The listing builds one solid part. Answer for the finished solid, in the listing's coordinates (mm). A direction names the side the tool comes from. Give positions to 0.01 mm unless a question says otherwise; leave off trailing zeros. Order: outer loops, then holes, each group sorted by start corner. A loop starts at its lowest first (then second) coordinate and runs counter-clockwise, first axis right, second up. Notation, with made-up numbers: (43, 85) - (90, 85) arc R15 cw to (90, 96) - close; hole circle Ø10 at (-14.75, 7.5). An arc over 180 degrees is marked (long way). Answer in a Markdown table with one row per item.
from build123d import *

# Parameters (mm, degrees)
SKETCH073_W             = 75.5
SKETCH073_H             = 44
PAD038_DEPTH            = 1
SKETCH074_W             = 15
SKETCH074_H             = 44
PAD039_DEPTH            = 9
SKETCH075_W             = 18
SKETCH075_H             = 44
PAD040_DEPTH            = 1
SKETCH076_W             = 10.5
SKETCH076_H             = 39.5
PAD041_DEPTH            = 30.5
SKETCH077_W             = 7
SKETCH077_H             = 30
POCKET027_DEPTH         = 39
SKETCH078_W             = 15
SKETCH078_H             = 6
POCKET028_DEPTH         = 15
SKETCH079_W             = 1.5
SKETCH079_H             = 44
PAD042_DEPTH            = 2
CHAMFER044_SIZE         = 1.2
FILLET011_R             = 7.5
CHAMFER045_SIZE         = 0.5
CHAMFER050_SIZE         = 0.3
BODY014_PLACEMENT_ANGLE = 180


with BuildPart() as part:
    # Sketch073 → Pad038 (new body)
    with BuildSketch(Plane.XY):
        with Locations((-30.25, 0)):
            Rectangle(SKETCH073_W, SKETCH073_H)
    extrude(amount=-PAD038_DEPTH)

    # Sketch074 (on Face5 of Pad038) → Pad039 (join)
    with BuildSketch(Plane.XY):
        Rectangle(SKETCH074_W, SKETCH074_H)
    extrude(amount=PAD039_DEPTH)

    # Sketch075 (on Face5 of Pad039) → Pad040 (join)
    with BuildSketch(Plane.XY.offset(9)):
        with Locations((-1.5, 0)):
            Rectangle(SKETCH075_W, SKETCH075_H)
    extrude(amount=PAD040_DEPTH)

    # Sketch076 (on Face7 of Pad040) → Pad041 (join)
    with BuildSketch(Plane.XY.offset(10)):
        Rectangle(SKETCH076_W, SKETCH076_H)
    extrude(amount=PAD041_DEPTH)

    # Sketch077 (on Face15 of Pad041) → Pocket027 (cut)
    with BuildSketch(Plane.XY.offset(40.5)):
        Rectangle(SKETCH077_W, SKETCH077_H)
    extrude(amount=-POCKET027_DEPTH, mode=Mode.SUBTRACT)

    # Sketch078 (on Face6 of Pocket027) → Pocket028 (cut)
    with BuildSketch(Plane.YZ.offset(7.5)):
        with Locations((0, 4.5)):
            Rectangle(SKETCH078_W, SKETCH078_H)
    extrude(amount=-POCKET028_DEPTH, mode=Mode.SUBTRACT)

    # Sketch079 (on Face4 of Pocket028) → Pad042 (join)
    with BuildSketch(Plane.XY):
        with Locations((-61.25, 0)):
            Rectangle(SKETCH079_W, SKETCH079_H)
    extrude(amount=PAD042_DEPTH)

    # Chamfer044
    chamfer044_edges = [part.edges().sort_by_distance(p)[0] for p in [
        (-62, 0, 2),
    ]]
    chamfer(chamfer044_edges, length=CHAMFER044_SIZE)

    # Fillet011
    fillet011_edges = [part.edges().sort_by_distance(p)[0] for p in [
        (0, 15, 1.5),
        (0, -15, 1.5),
    ]]
    fillet(fillet011_edges, radius=FILLET011_R)

    # Chamfer045
    chamfer045_edges = [part.edges().sort_by_distance(p)[0] for p in [
        (-7.5, 7.5, 4.5),
        (-7.5, 0, 7.5),
        (-7.5, -7.5, 4.5),
        (-7.5, 0, 1.5),
        (7.5, 7.5, 4.5),
        (7.5, 0, 1.5),
        (7.5, -7.5, 4.5),
        (7.5, 0, 7.5),
        (7.5, -22, 4.5),
        (7.5, 22, 4.5),
        (7.5, 0, -1),
        (-7.5, -22, 4.5),
        (-30.25, -22, -1),
        (-68, 0, -1),
        (-30.25, 22, -1),
        (-7.5, 22, 4.5),
        (-10.5, -22, 9.5),
        (-10.5, 22, 9.5),
    ]]
    chamfer(chamfer045_edges, length=CHAMFER045_SIZE)

    # Chamfer050
    chamfer050_edges = [part.edges().sort_by_distance(p)[0] for p in [
        (5.25, 19.75, 25.25),
        (-5.25, 19.75, 25.25),
        (-5.25, -19.75, 25.25),
        (5.25, -19.75, 25.25),
        (0, 19.75, 40.5),
        (-5.25, 0, 40.5),
        (5.25, 0, 40.5),
        (0, -19.75, 40.5),
        (-3.5, 0, 40.5),
        (0, -15, 40.5),
        (3.5, 0, 40.5),
        (0, 15, 40.5),
    ]]
    chamfer(chamfer050_edges, length=CHAMFER050_SIZE)


with BuildPart() as part_1:
    # Body014 placement: moved
    add(part.part.moved(Location((-106.5, -22, -136))).rotate(Axis((-106.5, -22, -136), (0, 0, 1)), BODY014_PLACEMENT_ANGLE))


solid = part_1.part
Item 1: Determine the mould class of faces 1 (the face through (-101.25, -22, -111)), 2 (the face through (-101, 0, -132)), 3 (the face through (-46, -22, -135)) for opening direction X: pulls with the +X half, pulls with the -X half, needs draft (parallel to the pull), parting line crosses it, or undercut.
Answer block:
| item | result |
|---|---|
| face 1 | pulls with the +X half |
| face 2 | needs draft |
| face 3 | undercut |
Item 2: Find section A-A on z = -99. Write down the section's boundary in (x, y), then the cut area to 3 significant figures.
Answer block:
| item | result |
|---|---|
| outline | (-111.75, -41.45) - (-111.45, -41.75) - (-101.55, -41.75) - (-101.25, -41.45) - (-101.25, -2.55) - (-101.55, -2.25) - (-111.45, -2.25) - (-111.75, -2.55) - close; hole (-110, -37) - (-103, -37) - (-103, -7) - (-110, -7) - close |
| area | 205 mm² |
Item 3: Consider line 1 (Y direction, x = -106.5, z = -117); line 2 (X direction, y = -25.5, z = -125); line 3 (Z direction, x = -54.5, y = -8). Determine where each line is inside the solid, lowest interval first.
Answer block:
| item | result |
|---|---|
| line 1 | -41.75 to -37, -7 to -2.25 |
| line 2 | -111.75 to -110, -103 to -101.25 |
| line 3 | -137 to -136 |
Item 4: Find section D-D on y = -40. Write down the section's boundary in (x, z), then the cut area to 3 significant figures.
Answer block:
| item | result |
|---|---|
| outline | (-114, -136.5) - (-113.5, -137) - (-39, -137) - (-38.5, -136.5) - (-38.5, -136) - (-44.5, -136) - (-44.5, -135.2) - (-45.7, -134) - (-46, -134) - (-46, -136) - (-99, -136) - (-99, -127) - (-96, -127) - (-96, -126) - (-101.25, -126) - (-101.25, -95.8) - (-101.55, -95.5) - (-111.45, -95.5) - (-111.75, -95.8) - (-111.75, -126) - (-114, -126) - close |
| area | 551 mm² |
Item 5: Each of these flat-tipped pins is pushed along its axis until it touches: P1, Ø12, axis at y = -20, z = -126.5, coming from the +X side; P2, Ø4, axis at x = -54.5, y = -19, coming from the +Z side; P3, Ø5, axis at y = -15, z = -107, coming from the -X side; P4, Ø20, axis at x = -104, y = -16, coming from the +Z side. Where does it stop, or does it pass through?
Answer block:
| item | result |
|---|---|
| P1 | x = -96 |
| P2 | z = -136 |
| P3 | x = -111.75 |
| P4 | z = -95.5 |
Item 6: Which of the six approach directions +Z, -Z, +X, -X, +Y, -Y give full straight-line access (tool end or side, diameter ignored) to faces 4 (the face through (-103, -22, -115)), 5 (the face through (-106, -2.25, -111)), 6 (the face through (-99, -21.7, -135.6)), 7 (the face through (-101, -22, -128.5)), 8 (the face through (-107, -22, -134.5))?
Answer block:
| item | result |
|---|---|
| face 4 | +Z |
| face 5 | +Z, +X, -X, +Y |
| face 6 | +Y, -Y |
| face 7 | +X, -X |
| face 8 | -X |
Item 7: Find section B-B on y = -23. Count the separate pieces of the cut face and the enclosed holes in it, then the cut area to 3 significant figures.
Answer block:
| item | result |
|---|---|
| separate pieces | 3 |
| enclosed holes | 0 |
| area | 229 mm² |
Item 8: Find section C-C on x = -104. Write down the section's boundary in (y, z), then the cut area to 3 significant figures.
Answer block:
| item | result |
|---|---|
| outline | (-44, -136.5) - (-43.5, -137) - (-0.5, -137) - (0, -136.5) - (0, -126) - (-2.25, -126) - (-2.25, -95.8) - (-2.55, -95.5) - (-6.7, -95.5) - (-7, -95.8) - (-7, -127) arc R7.5 cw to (-14.5, -134.5) - (-29.5, -134.5) arc R7.5 cw to (-37, -127) - (-37, -95.8) - (-37.3, -95.5) - (-41.45, -95.5) - (-41.75, -95.8) - (-41.75, -126) - (-44, -126) - close |
| area | 542 mm² |
